Check sheet for the modelled part. Datum: model origin and axes. Units: mm. Face numbers are marked on the shaded views. Coordinates: 2 decimals unless noted, no trailing zeros. Loops run counter-clockwise (first coordinate to the right, second up) from the corner with the lowest first, then second, coordinate; pieces in that order, holes last.
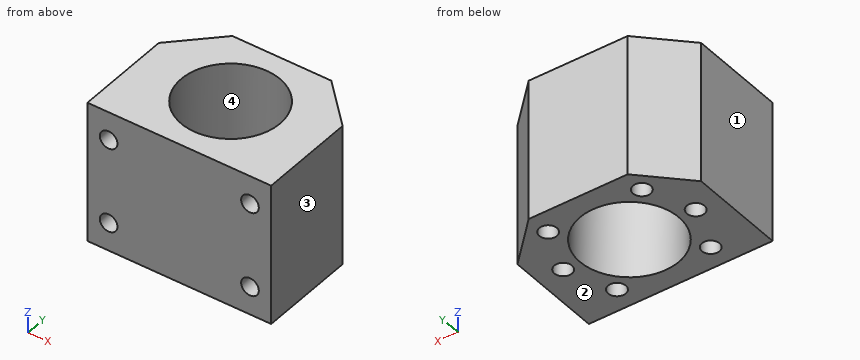
```python
from build123d import *

# Parameters (mm, degrees)
SKETCH1_W           = 52
SKETCH1_H           = 39.5
SKETCH1_R           = 2.5
SKETCH1_R_2         = 14
BOSS_EXTRUDE1_DEPTH = 40
CHAMFER1_SIZE       = 12
SKETCH1_3_R         = 2.5
CUT_EXTRUDE1_DEPTH  = 16.5
SKETCH2_R           = 2.5
CUT_EXTRUDE2_DEPTH  = 8


with BuildPart() as part:
    # Sketch1 → Boss-Extrude1 (new body)
    with BuildSketch(Plane.XY):
        Rectangle(SKETCH1_W, SKETCH1_H)
        with Locations((13.258252147, 13.258252147)):
            Circle(SKETCH1_R, mode=Mode.SUBTRACT)
        with Locations((-13.258252147, 13.258252147)):
            Circle(SKETCH1_R, mode=Mode.SUBTRACT)
        with Locations((-18.75, 0)):
            Circle(SKETCH1_R, mode=Mode.SUBTRACT)
        with Locations((-13.258252147, -13.258252147)):
            Circle(SKETCH1_R, mode=Mode.SUBTRACT)
        with Locations((13.258252147, -13.258252147)):
            Circle(SKETCH1_R, mode=Mode.SUBTRACT)
        with Locations((18.75, 0)):
            Circle(SKETCH1_R, mode=Mode.SUBTRACT)
        Circle(SKETCH1_R_2, mode=Mode.SUBTRACT)
        with Locations((13.258252147, -13.258252147)):
            Circle(SKETCH1_R)
        with Locations((-13.258252147, -13.258252147)):
            Circle(SKETCH1_R)
        with Locations((-18.75, 0)):
            Circle(SKETCH1_R)
        with Locations((18.75, 0)):
            Circle(SKETCH1_R)
        with Locations((-13.258252147, 13.258252147)):
            Circle(SKETCH1_R)
        with Locations((13.258252147, 13.258252147)):
            Circle(SKETCH1_R)
    extrude(amount=BOSS_EXTRUDE1_DEPTH)

    # Chamfer1
    chamfer1_edges = [part.edges().sort_by_distance(p)[0] for p in [
        (-26, 19.75, 20),
        (26, 19.75, 20),
    ]]
    chamfer(chamfer1_edges, length=CHAMFER1_SIZE)

    # Sketch1<3> → Cut-Extrude1 (cut)
    with BuildSketch(Plane.XY):
        with Locations((13.258252147, 13.258252147)):
            Circle(SKETCH1_3_R)
        with Locations((18.75, 0)):
            Circle(SKETCH1_3_R)
        with Locations((13.258252147, -13.258252147)):
            Circle(SKETCH1_3_R)
        with Locations((-13.258252147, -13.258252147)):
            Circle(SKETCH1_3_R)
        with Locations((-18.75, 0)):
            Circle(SKETCH1_3_R)
        with Locations((-13.258252147, 13.258252147)):
            Circle(SKETCH1_3_R)
    extrude(amount=CUT_EXTRUDE1_DEPTH, mode=Mode.SUBTRACT)

    # Sketch2 → Cut-Extrude2 (cut)
    with BuildSketch(Plane.XZ.offset(19.75)):
        with Locations(Location((20, 8, 0), (0, 0, 270))):
            Circle(SKETCH2_R)
        with Locations(Location((-20, 8, 0), (0, 0, 270))):
            Circle(SKETCH2_R)
        with Locations(Location((20, 32, 0), (0, 0, 270))):
            Circle(SKETCH2_R)
        with Locations(Location((-20, 32, 0), (0, 0, 270))):
            Circle(SKETCH2_R)
    extrude(amount=-CUT_EXTRUDE2_DEPTH, mode=Mode.SUBTRACT)


solid = part.part
```
1) Scan lines: line 1 (X direction, y = -16.75, z = 8); line 2 (X direction, y = -14.5, z = 8); line 3 (Y direction, x = -12, z = 12.5). Record each from-to range of solid material in increasing order.
Answer sheet:
line 1: x = -26 to -22.5, -17.5 to 17.5, 22.5 to 26
line 2: x = -26 to -22.5, -17.5 to -15.43, -11.09 to 11.09, 15.43 to 17.5, 22.5 to 26
line 3: y = -19.75 to -15.42, -11.1 to -7.21, 7.21 to 11.1, 15.42 to 19.75
2) Section check C-C on z = 32. Enter the section's corners in (x, y).
Answer sheet:
outline: (-26, -19.75) - (-22.5, -19.75) - (-22.5, -11.75) - (-17.5, -11.75) - (-17.5, -19.75) - (17.5, -19.75) - (17.5, -11.75) - (22.5, -11.75) - (22.5, -19.75) - (26, -19.75) - (26, 7.75) - (14, 19.75) - (-14, 19.75) - (-26, 7.75) - close; hole circle Ø28 at (0, 0)
3) Section check A-A on y = 0. Enter the section's corners in (x, z), plus the area to 3 significant figures.
Answer sheet:
outline: (-26, 0) - (-21.25, 0) - (-21.25, 16.5) - (-16.25, 16.5) - (-16.25, 0) - (-14, 0) - (-14, 40) - (-26, 40) - close; (14, 0) - (16.25, 0) - (16.25, 16.5) - (21.25, 16.5) - (21.25, 0) - (26, 0) - (26, 40) - (14, 40) - close
area: 795 mm2
4) Section check B-B on x = 0. Enter the section's corners in (y, z), plus the area to 3 significant figures.
Answer sheet:
outline: (-19.75, 0) - (-14, 0) - (-14, 40) - (-19.75, 40) - close; (14, 0) - (19.75, 0) - (19.75, 40) - (14, 40) - close
area: 460 mm2
5) Mould release check, pull along X, two halves, no side actions. Record for the marked faces 1, 2, 3 and 4: +X half, -X half, draft (parallel to the pull), parting line (faces both ways), or undercut.
Answer sheet:
face 1: -X half
face 2: draft
face 3: +X half
face 4: undercut
6) Section check D-D on z = 7. Enter the section's corners in (x, y), plus the area to 3 significant figures.
Answer sheet:
outline: (-26, -19.75) - (-22.29, -19.75) - (-22.29, -11.75) - (-17.71, -11.75) - (-17.71, -19.75) - (17.71, -19.75) - (17.71, -11.75) - (22.29, -11.75) - (22.29, -19.75) - (26, -19.75) - (26, 7.75) - (14, 19.75) - (-14, 19.75) - (-26, 7.75) - close; hole circle Ø5 at (-18.75, 0); hole circle Ø5 at (-13.26, -13.26); hole circle Ø5 at (-13.26, 13.26); hole circle Ø28 at (0, 0); hole circle Ø5 at (13.26, -13.26); hole circle Ø5 at (13.26, 13.26); hole circle Ø5 at (18.75, 0)
area: 1,100 mm2
7) Depth check by flat-ended pin: pin 1 (4 mm diameter, centred on x = -18.75, y = 0, fed in from -Z); pin 2 (1.5 mm diameter, centred on x = 20.5, z = 9, fed in from -Y); pin 3 (4 mm diameter, centred on y = 15, z = 28, fed in from +X). Enter the tip coordinate at first touch or a pass-through.
Answer sheet:
pin 1: stops at z = 16.5
pin 2: stops at y = -11.75
pin 3: stops at x = 20.75
